Autodesk Inventor part; units mm, degrees
ref_plane "YZ Plane" through (0, 0, 0) normal (1, 0, 0) x (0, 1, 0)
ref_plane "XZ Plane" through (0, 0, 0) normal (0, 1, 0) x (-1, 0, 0)
ref_plane "XY Plane" through (0, 0, 0) normal (0, 0, 1) x (1, 0, 0)
sketch "Sketch1" plane through (0, 0, 0) normal (0, 0, 1) x (1, 0, 0)
  circle A0 centre (0, 0) radius 7.5
  dimension "d0" = 15
extrude "Extrusion1" add sketch "Sketch1" along normal blind 15
hole "Hole1" at (0, 0, 15) direction (0, 0, -1) diameter 2.4 end through all
sketch "Sketch3" plane through (0, 0, 15) normal (0, 0, 1) x (1, 0, 0)
  circle A0 centre (0, 0) radius 1.2
  circle A1 centre (0, 0) radius 7.5
  circle A2 centre (0, 0) radius 1.9
  dimension "d16" = 3.8
extrude "Extrusion3" cut sketch "Sketch3" against normal blind 0.5 contours A2
sketch "Sketch2" plane through (0, 0, 15) normal (0, 0, 1) x (1, 0, 0)
  circle A0 centre (0, 0) radius 1.2
  circle A1 centre (-3.5, 0) radius 0.75
  dimension "d12" = 1.5
  dimension "d13" = 3.5
extrude "Extrusion2" cut sketch "Sketch2" against normal through all contours A1
properties part number "Jig_Bearing_OD_Asm"
Work out the finished part from the listing and answer in its coordinate system (mm). A direction names the side the tool comes from. Coordinates: 2 decimals unless noted, no trailing zeros. Order: outer loops, then holes, each group sorted by start corner. A loop starts at its lowest first (then second) coordinate and runs counter-clockwise, first axis right, second up. Notation, with made-up numbers: (40.5, 27.25) - (93.5, 27.25) arc R9 ccw to (93.5, 41.25) - close; hole circle Ø10 at (-21.5, -35). An arc over 180 degrees is marked (long way). Put each result on its own line as item: value. Start each with the question number.
1) Find section B-B (x = -3.5). Give the vertices of the cut face in (y, z), plus the area to 3 significant figures.
2) Find section D-D (y = -1.5). Give the vertices of the cut face in (x, z), plus the area to 3 significant figures.
3) Find section A-A (y = 0). Give the vertices of the cut face in (x, z), plus the area to 3 significant figures.
4) For a pull along X with two mould halves and no side action, classify faces 3 (the flat face through (-1, 1, 14.5)), 4 (the cylindrical face through (-7.493, -0.33, 7.395)), 5 (the flat face through (2, 0, 0)) as released by +X, released by -X, zero draft, split by the parting line, or undercut.
5) Find the intervals of material crossed by line 1 (Y direction, x = 0, z = 14.85); line 2 (Y direction, x = 0, z = 11.5); line 3 (X direction, y = 2.25, z = 11), in increasing order. Write a range as from..to.
6) Flat-ended cylindrical pins translate along their axes: pin 1 (1 mm diameter, centred on y = 2.5, z = 12, fed in from +X); pin 2 (5 mm diameter, centred on y = -4.5, z = 3, fed in from -X); pin 3 (8 mm diameter, centred on y = 5, z = 6, fed in from +X). Find the tip coordinate at first contact, or state that the pin passes through.
7) Find section C-C (z = 12). Give the vertices of the cut face in (x, y).
8) For faces 1 (the cylindrical face through (-1.9, 0.08, 14.75)), 2 (the cylindrical face through (-1.01, -0.65, 7.15)), determine the directions among +Z, -Z, +X, -X, +Y, -Y from which every point of the face is accessible in a straight line to the end or side of a thin tool.
Results list:
1. outline: (-6.63, 0) - (-0.75, 0) - (-0.75, 15) - (-6.63, 15) - close; (0.75, 0) - (6.63, 0) - (6.63, 15) - (0.75, 15) - close
1. area: 176 mm^2
2. outline: (-7.35, 0) - (7.35, 0) - (7.35, 15) - (1.17, 15) - (1.17, 14.5) - (-1.17, 14.5) - (-1.17, 15) - (-7.35, 15) - close
2. area: 219 mm^2
3. outline: (-7.5, 0) - (-4.25, 0) - (-4.25, 15) - (-7.5, 15) - close; (-2.75, 0) - (-1.2, 0) - (-1.2, 14.5) - (-1.9, 14.5) - (-1.9, 15) - (-2.75, 15) - close; (1.2, 0) - (7.5, 0) - (7.5, 15) - (1.9, 15) - (1.9, 14.5) - (1.2, 14.5) - close
3. area: 166 mm^2
4. face 3: undercut
4. face 4: split by the parting line
4. face 5: zero draft
5. line 1: y = -7.5..-1.9, 1.9..7.5
5. line 2: y = -7.5..-1.2, 1.2..7.5
5. line 3: x = -7.15..7.15
6. pin 1: stops at x = 7.23
6. pin 2: stops at x = -7.23
6. pin 3: stops at x = 7.43
7. outline: circle Ø15 at (0, 0); hole circle Ø1.5 at (-3.5, 0); hole circle Ø2.4 at (0, 0)
8. face 1: +Z
8. face 2: +Z, -Z
